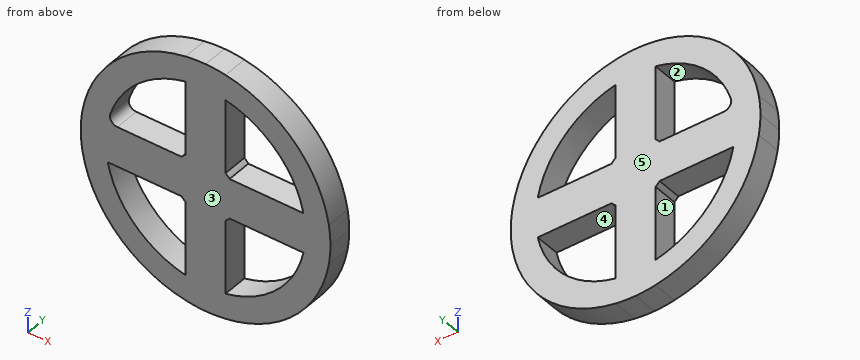
from build123d import *

# Parameters (mm, degrees)
F1_DEPTH = 10
F3_DEPTH = 10
F4_R     = 5.005299482
F5_DEPTH = 10
F6_R     = 3


with BuildPart() as f1:
    # F0 (on Front) → F1 (new body)
    with BuildSketch(Plane.XZ):
        with BuildLine():
            Line((-8, 39.1918358845), (-8, 49.355850717))
            ThreePointArc((-8, 49.355850717), (-35.3553390593, 35.3553390593), (-49.355850717, 8))
            Line((-49.355850717, 8), (-39.1918358845, 8))
            ThreePointArc((-39.1918358845, 8), (-28.2842712475, 28.2842712475), (-8, 39.1918358845))
        make_face()
        with BuildLine():
            Line((8, -8), (8, 0))
            Line((8, 0), (5, 0))
            ThreePointArc((5, 0), (3.5355339059, -3.5355339059), (0, -5))
            Line((0, -5), (0, -8))
            Line((0, -8), (8, -8))
        make_face()
        with BuildLine():
            ThreePointArc((8, -9.6046863561), (8.8388347648, -8.8388347648), (9.6046863561, -8))
            Line((9.6046863561, -8), (8, -8))
            Line((8, -8), (8, -9.6046863561))
        make_face()
        with BuildLine():
            ThreePointArc((9.6046863561, -8), (11.7539052968, -4.2539052968), (12.5, 0))
            Line((12.5, 0), (8, 0))
            Line((8, 0), (8, -8))
            Line((8, -8), (9.6046863561, -8))
        make_face()
        with BuildLine():
            ThreePointArc((-8, -9.6046863561), (-4.2539052968, -11.7539052968), (0, -12.5))
            Line((0, -12.5), (0, -8))
            Line((0, -8), (-8, -8))
            Line((-8, -8), (-8, -9.6046863561))
        make_face()
        with BuildLine():
            Line((5, 0), (8, 0))
            Line((8, 0), (8, 8))
            Line((8, 8), (0, 8))
            Line((0, 8), (0, 5))
            ThreePointArc((0, 5), (3.5355339059, 3.5355339059), (5, 0))
        make_face()
        with BuildLine():
            Line((8, 0), (12.5, 0))
            ThreePointArc((12.5, 0), (11.7539052968, 4.2539052968), (9.6046863561, 8))
            Line((9.6046863561, 8), (8, 8))
            Line((8, 8), (8, 0))
        make_face()
        with BuildLine():
            Line((12.5, 0), (40, 0))
            ThreePointArc((40, 0), (39.7974461202, 4.0203584802), (39.1918358845, 8))
            Line((39.1918358845, 8), (9.6046863561, 8))
            ThreePointArc((9.6046863561, 8), (11.7539052968, 4.2539052968), (12.5, 0))
        make_face()
        with BuildLine():
            ThreePointArc((0, -12.5), (4.2539052968, -11.7539052968), (8, -9.6046863561))
            Line((8, -9.6046863561), (8, -8))
            Line((8, -8), (0, -8))
            Line((0, -8), (0, -12.5))
        make_face()
        with BuildLine():
            ThreePointArc((-9.6046863561, -8), (-8.8388347648, -8.8388347648), (-8, -9.6046863561))
            Line((-8, -9.6046863561), (-8, -8))
            Line((-8, -8), (-9.6046863561, -8))
        make_face()
        with BuildLine():
            Line((-8, -8), (0, -8))
            Line((0, -8), (0, -5))
            ThreePointArc((0, -5), (-3.5355339059, -3.5355339059), (-5, 0))
            Line((-5, 0), (-8, 0))
            Line((-8, 0), (-8, -8))
        make_face()
        with BuildLine():
            Line((-9.6046863561, -8), (-8, -8))
            Line((-8, -8), (-8, 0))
            Line((-8, 0), (-12.5, 0))
            ThreePointArc((-12.5, 0), (-11.7539052968, -4.2539052968), (-9.6046863561, -8))
        make_face()
        with BuildLine():
            Line((0, 5), (0, 8))
            Line((0, 8), (-8, 8))
            Line((-8, 8), (-8, 0))
            Line((-8, 0), (-5, 0))
            ThreePointArc((-5, 0), (-3.5355339059, 3.5355339059), (0, 5))
        make_face()
        with BuildLine():
            Line((-8, 0), (-8, 8))
            Line((-8, 8), (-9.6046863561, 8))
            ThreePointArc((-9.6046863561, 8), (-11.7539052968, 4.2539052968), (-12.5, 0))
            Line((-12.5, 0), (-8, 0))
        make_face()
        with BuildLine():
            Line((-8, 8), (-8, 9.6046863561))
            ThreePointArc((-8, 9.6046863561), (-8.8388347648, 8.8388347648), (-9.6046863561, 8))
            Line((-9.6046863561, 8), (-8, 8))
        make_face()
        with BuildLine():
            Line((0, 8), (0, 12.5))
            ThreePointArc((0, 12.5), (-4.2539052968, 11.7539052968), (-8, 9.6046863561))
            Line((-8, 9.6046863561), (-8, 8))
            Line((-8, 8), (0, 8))
        make_face()
        with BuildLine():
            Line((8, 8), (8, 9.6046863561))
            ThreePointArc((8, 9.6046863561), (4.2539052968, 11.7539052968), (0, 12.5))
            Line((0, 12.5), (0, 8))
            Line((0, 8), (8, 8))
        make_face()
        with BuildLine():
            Line((8, 8), (9.6046863561, 8))
            ThreePointArc((9.6046863561, 8), (8.8388347648, 8.8388347648), (8, 9.6046863561))
            Line((8, 9.6046863561), (8, 8))
        make_face()
        with BuildLine():
            ThreePointArc((39.1918358845, -8), (39.7974461202, -4.0203584802), (40, 0))
            Line((40, 0), (12.5, 0))
            ThreePointArc((12.5, 0), (11.7539052968, -4.2539052968), (9.6046863561, -8))
            Line((9.6046863561, -8), (39.1918358845, -8))
        make_face()
        with BuildLine():
            Line((-9.6046863561, 8), (-39.1918358845, 8))
            ThreePointArc((-39.1918358845, 8), (-39.7974461202, 4.0203584802), (-40, 0))
            Line((-40, 0), (-12.5, 0))
            ThreePointArc((-12.5, 0), (-11.7539052968, 4.2539052968), (-9.6046863561, 8))
        make_face()
        with BuildLine():
            ThreePointArc((-40, 0), (-39.7974461202, -4.0203584802), (-39.1918358845, -8))
            Line((-39.1918358845, -8), (-9.6046863561, -8))
            ThreePointArc((-9.6046863561, -8), (-11.7539052968, -4.2539052968), (-12.5, 0))
            Line((-12.5, 0), (-40, 0))
        make_face()
        with BuildLine():
            Line((0, 12.5), (0, 40))
            ThreePointArc((0, 40), (-4.0203584802, 39.7974461202), (-8, 39.1918358845))
            Line((-8, 39.1918358845), (-8, 9.6046863561))
            ThreePointArc((-8, 9.6046863561), (-4.2539052968, 11.7539052968), (0, 12.5))
        make_face()
        with BuildLine():
            Line((8, 9.6046863561), (8, 39.1918358845))
            ThreePointArc((8, 39.1918358845), (4.0203584802, 39.7974461202), (0, 40))
            Line((0, 40), (0, 12.5))
            ThreePointArc((0, 12.5), (4.2539052968, 11.7539052968), (8, 9.6046863561))
        make_face()
        with BuildLine():
            ThreePointArc((-8, -39.1918358845), (-4.0203584802, -39.7974461202), (0, -40))
            Line((0, -40), (0, -12.5))
            ThreePointArc((0, -12.5), (-4.2539052968, -11.7539052968), (-8, -9.6046863561))
            Line((-8, -9.6046863561), (-8, -39.1918358845))
        make_face()
        with BuildLine():
            ThreePointArc((0, -40), (4.0203584802, -39.7974461202), (8, -39.1918358845))
            Line((8, -39.1918358845), (8, -9.6046863561))
            ThreePointArc((8, -9.6046863561), (4.2539052968, -11.7539052968), (0, -12.5))
            Line((0, -12.5), (0, -40))
        make_face()
        with BuildLine():
            ThreePointArc((-49.355850717, -8), (-35.3553390593, -35.3553390593), (-8, -49.355850717))
            Line((-8, -49.355850717), (-8, -39.1918358845))
            ThreePointArc((-8, -39.1918358845), (-28.2842712475, -28.2842712475), (-39.1918358845, -8))
            Line((-39.1918358845, -8), (-49.355850717, -8))
        make_face()
        with BuildLine():
            Line((-39.1918358845, 8), (-49.355850717, 8))
            ThreePointArc((-49.355850717, 8), (-49.8387025105, 4.0129455609), (-50, 0))
            Line((-50, 0), (-40, 0))
            ThreePointArc((-40, 0), (-39.7974461202, 4.0203584802), (-39.1918358845, 8))
        make_face()
        with BuildLine():
            ThreePointArc((-50, 0), (-49.8387025105, -4.0129455609), (-49.355850717, -8))
            Line((-49.355850717, -8), (-39.1918358845, -8))
            ThreePointArc((-39.1918358845, -8), (-39.7974461202, -4.0203584802), (-40, 0))
            Line((-40, 0), (-50, 0))
        make_face()
        with BuildLine():
            Line((0, 40), (0, 50))
            ThreePointArc((0, 50), (-4.0129455609, 49.8387025105), (-8, 49.355850717))
            Line((-8, 49.355850717), (-8, 39.1918358845))
            ThreePointArc((-8, 39.1918358845), (-4.0203584802, 39.7974461202), (0, 40))
        make_face()
        with BuildLine():
            Line((8, 39.1918358845), (8, 49.355850717))
            ThreePointArc((8, 49.355850717), (4.0129455609, 49.8387025105), (0, 50))
            Line((0, 50), (0, 40))
            ThreePointArc((0, 40), (4.0203584802, 39.7974461202), (8, 39.1918358845))
        make_face()
        with BuildLine():
            Line((39.1918358845, 8), (49.355850717, 8))
            ThreePointArc((49.355850717, 8), (35.3553390593, 35.3553390593), (8, 49.355850717))
            Line((8, 49.355850717), (8, 39.1918358845))
            ThreePointArc((8, 39.1918358845), (28.2842712475, 28.2842712475), (39.1918358845, 8))
        make_face()
        with BuildLine():
            Line((40, 0), (50, 0))
            ThreePointArc((50, 0), (49.8387025105, 4.0129455609), (49.355850717, 8))
            Line((49.355850717, 8), (39.1918358845, 8))
            ThreePointArc((39.1918358845, 8), (39.7974461202, 4.0203584802), (40, 0))
        make_face()
        with BuildLine():
            ThreePointArc((49.355850717, -8), (49.8387025105, -4.0129455609), (50, 0))
            Line((50, 0), (40, 0))
            ThreePointArc((40, 0), (39.7974461202, -4.0203584802), (39.1918358845, -8))
            Line((39.1918358845, -8), (49.355850717, -8))
        make_face()
        with BuildLine():
            ThreePointArc((8, -49.355850717), (35.3553390593, -35.3553390593), (49.355850717, -8))
            Line((49.355850717, -8), (39.1918358845, -8))
            ThreePointArc((39.1918358845, -8), (28.2842712475, -28.2842712475), (8, -39.1918358845))
            Line((8, -39.1918358845), (8, -49.355850717))
        make_face()
        with BuildLine():
            ThreePointArc((-8, -49.355850717), (-4.0129455609, -49.8387025105), (0, -50))
            Line((0, -50), (0, -40))
            ThreePointArc((0, -40), (-4.0203584802, -39.7974461202), (-8, -39.1918358845))
            Line((-8, -39.1918358845), (-8, -49.355850717))
        make_face()
        with BuildLine():
            ThreePointArc((0, -50), (4.0129455609, -49.8387025105), (8, -49.355850717))
            Line((8, -49.355850717), (8, -39.1918358845))
            ThreePointArc((8, -39.1918358845), (4.0203584802, -39.7974461202), (0, -40))
            Line((0, -40), (0, -50))
        make_face()
    extrude(amount=F1_DEPTH)

    # F2 (on face) → F3 (join)
    with BuildSketch(Plane.XZ.offset(10)):
        with BuildLine():
            Line((7.6082753949, 1.9267198172), (4.613865055, 1.9267198172))
            ThreePointArc((4.613865055, 1.9267198172), (4.9025159498, 0.9825158332), (5, 0))
            ThreePointArc((5, 0), (4.9024071863, -0.9830583809), (4.6134384879, -1.9277409883))
            Line((4.6134384879, -1.9277409883), (7.6082753949, -1.9277409883))
            Line((7.6082753949, -1.9277409883), (7.6082753949, 0))
            Line((7.6082753949, 0), (7.6082753949, 1.9267198172))
        make_face()
        with BuildLine():
            ThreePointArc((5, 0), (4.9025159498, 0.9825158332), (4.613865055, 1.9267198172))
            ThreePointArc((4.613865055, 1.9267198172), (-4.9999999694, 0.0005533421), (4.6134384879, -1.9277409883))
            ThreePointArc((4.6134384879, -1.9277409883), (4.9024071863, -0.9830583809), (5, 0))
        make_face()
    extrude(amount=-F3_DEPTH)

    # F4 (on face) → F5 (join)
    with BuildSketch(Plane.XZ.offset(10)):
        Circle(F4_R)
    extrude(amount=-F5_DEPTH)

    # F6
    f6_edges = [f1.edges().sort_by_distance(p)[0] for p in [
        (-39.191836, -5, 8),
    ]]
    fillet(f6_edges, radius=F6_R)


solid = f1.part
Verification items for the finished model (mm, model axes). Face numbers are marked on the shaded views. A direction names the side the tool comes from. Coordinates: 2 decimals unless noted, no trailing zeros. Order: outer loops, then holes, each group sorted by start corner. A loop starts at its lowest first (then second) coordinate and runs counter-clockwise, first axis right, second up. Notation, with made-up numbers: (8.25, 0.5) -> (26.25, 0.5) arc R23 ccw to (26.25, 8.5) -> close; hole circle Ø3 at (49.5, 10). An arc over 180 degrees is marked (long way). Put each result on its own line as item: value. Start each with the question number.
1. Cross-section at C-C, the plane x = 16.5. Record the boundary of the cut face in (y, z), then the cut area to 3 significant figures.
2. Material ranges on L1, parallel to X at y = -8.5, z = 23.5; L2, parallel to X at y = -5.75, z = 34; L3, parallel to Z at x = 13.5, y = -2.5, recorded low to high. Write a range as [from, to].
3. Go/stop test with flat-tipped pins: pin 1 Ø1 at (y, z) = (-5.5, -38) entering from +X; pin 2 Ø5 at (x, y) = (-24.5, -7.5) entering from -Z; pin 3 Ø5 at (y, z) = (-5.5, 22) entering from +X. Record where each tip stops, or that it passes through.
4. Cross-section at B-B, the plane z = -29. Record the boundary of the cut face in (x, y).
5. Cross-section at D-D, the plane x = 41. Record the boundary of the cut face in (y, z).
6. Cross-section at A-A, the plane y = -7. Record the boundary of the cut face in (x, z).
7. Access from +Z, -Z, +X, -X, +Y, -Y to the whole of each face (thin tool, end or side, straight path). Record for the marked faces 4 and 5.
8. Mould release check, pull along Z, two halves, no side actions. Record for the marked faces 1, 2 and 3: released by +Z, released by -Z, zero draft, split by the parting line, or undercut.
Computed:
1. outline: (-10, -47.2) -> (0, -47.2) -> (0, -36.44) -> (-10, -36.44) -> close; (-10, -8) -> (0, -8) -> (0, 8) -> (-10, 8) -> close; (-10, 36.44) -> (0, 36.44) -> (0, 47.2) -> (-10, 47.2) -> close
1. area: 375 mm2
2. L1: [-44.13, -32.37], [-8, 8], [32.37, 44.13]
2. L2: [-36.66, -21.07], [-8, 8], [21.07, 36.66]
2. L3: [-48.14, -37.65], [-8, 8], [37.65, 48.14]
3. pin 1: x = 33.07
3. pin 2: z = -44.9
3. pin 3: x = 46.04
4. outline: (-40.73, -10) -> (-27.55, -10) -> (-27.55, 0) -> (-40.73, 0) -> close; (-8, -10) -> (8, -10) -> (8, 0) -> (-8, 0) -> close; (27.55, -10) -> (40.73, -10) -> (40.73, 0) -> (27.55, 0) -> close
5. outline: (-10, -28.62) -> (0, -28.62) -> (0, 28.62) -> (-10, 28.62) -> close
6. outline: circle Ø100 at (0, 0); hole (-39.19, -8) arc R40 ccw to (-8, -39.19) -> (-8, -9.6) arc R12.5 cw to (-9.6, -8) -> close; hole (-38.19, 11.89) arc R3 ccw to (-35.33, 8) -> (-9.6, 8) arc R12.5 cw to (-8, 9.6) -> (-8, 39.19) arc R40 ccw to start; hole (8, -39.19) arc R40 ccw to (39.19, -8) -> (9.6, -8) arc R12.5 cw to (8, -9.6) -> close; hole (8, 9.6) arc R12.5 cw to (9.6, 8) -> (39.19, 8) arc R40 ccw to (8, 39.19) -> close
7. face 4: +Y, -Y
7. face 5: +Z, -Z, +X, -X, +Y
8. face 1: undercut
8. face 2: undercut
8. face 3: zero draft
